```python
from build123d import *

# Parameters (mm, degrees)
BOSS_EXTRUDE1_DEPTH = 9.525
SKETCH1_3_R         = 3.81
BOSS_EXTRUDE2_DEPTH = 2.54
FILLET1_R           = 2.54
SKETCH2_R           = 2.54
CUT_EXTRUDE1_DEPTH  = 106.176870727
SKETCH7_R           = 6.35
CUT_EXTRUDE2_DEPTH  = 18.415
FILLET2_R           = 2.54
FILLET3_R           = 2.54


with BuildPart() as part:
    # Sketch1 → Boss-Extrude1 (new, symmetric)
    with BuildSketch(Plane.XY):
        with BuildLine():
            ThreePointArc((61.722, 65.850540956), (66.416458594, 34.38975697), (39.6875, 17.145))
            Line((39.6875, 17.145), (39.6875, 0))
            Line((39.6875, 0), (79.375, 0))
            Line((79.375, 0), (79.375, 5.461))
            Line((79.375, 5.461), (49.2125, 5.461))
            Line((49.2125, 5.461), (49.2125, 13.012981804))
            ThreePointArc((49.2125, 13.012981804), (67.609880758, 25.71564604), (74.481791773, 46.99))
            ThreePointArc((74.481791773, 46.99), (72.157634164, 58.995640214), (65.823660173, 69.455940354))
            Line((65.823660173, 69.455940354), (61.722, 65.850540956))
        make_face()
        with BuildLine():
            Line((39.6875, 0), (39.6875, 17.145))
            ThreePointArc((39.6875, 17.145), (12.958541406, 34.38975697), (17.653, 65.850540956))
            Line((17.653, 65.850540956), (13.551339827, 69.455940354))
            ThreePointArc((13.551339827, 69.455940354), (7.217365836, 58.995640214), (4.893208227, 46.99))
            ThreePointArc((4.893208227, 46.99), (11.765119242, 25.71564604), (30.1625, 13.012981804))
            Line((30.1625, 13.012981804), (30.1625, 5.461))
            Line((30.1625, 5.461), (0, 5.461))
            Line((0, 5.461), (0, 0))
            Line((0, 0), (39.6875, 0))
        make_face()
    extrude(amount=BOSS_EXTRUDE1_DEPTH, both=True)

    # Sketch1<3> → Boss-Extrude2 (add, symmetric)
    # profile 1 of 2: a face of its own
    with BuildSketch(Plane.XY):
        with BuildLine():
            Line((0, 46.99), (0, 5.461))
            Line((0, 5.461), (30.1625, 5.461))
            Line((30.1625, 5.461), (30.1625, 13.012981804))
            ThreePointArc((30.1625, 13.012981804), (11.765119242, 25.71564604), (4.893208227, 46.99))
            Line((4.893208227, 46.99), (0, 46.99))
        make_face()
        with Locations((8.9535, 17.526)):
            Circle(SKETCH1_3_R, mode=Mode.SUBTRACT)
    # profile 2 of 2: a face of its own
    with BuildSketch(Plane.XY):
        with BuildLine():
            Line((49.2125, 5.461), (79.375, 5.461))
            Line((79.375, 5.461), (79.375, 46.99))
            Line((79.375, 46.99), (74.481791773, 46.99))
            ThreePointArc((74.481791773, 46.99), (67.609880758, 25.71564604), (49.2125, 13.012981804))
            Line((49.2125, 13.012981804), (49.2125, 5.461))
        make_face()
        with Locations((70.4215, 17.526)):
            Circle(SKETCH1_3_R, mode=Mode.SUBTRACT)
    extrude(amount=BOSS_EXTRUDE2_DEPTH, both=True)

    # Fillet1
    fillet1_edges = [part.edges().sort_by_distance(p)[0] for p in [
        (17.653, 65.850540956, 0),
    ]]
    fillet(fillet1_edges, radius=FILLET1_R)
    fillet1_2_edges = [part.edges().sort_by_distance(p)[0] for p in [
        (61.722, 65.850540956, 0),
    ]]
    fillet(fillet1_2_edges, radius=FILLET1_R)
    fillet1_3_edges = [part.edges().sort_by_distance(p)[0] for p in [
        (0, 2.7305, -9.525),
    ]]
    fillet(fillet1_3_edges, radius=FILLET1_R)
    fillet1_4_edges = [part.edges().sort_by_distance(p)[0] for p in [
        (79.375, 2.7305, -9.525),
    ]]
    fillet(fillet1_4_edges, radius=FILLET1_R)
    fillet1_5_edges = [part.edges().sort_by_distance(p)[0] for p in [
        (13.551339827, 69.455940354, 0),
    ]]
    fillet(fillet1_5_edges, radius=FILLET1_R)
    fillet1_6_edges = [part.edges().sort_by_distance(p)[0] for p in [
        (0, 2.7305, 9.525),
    ]]
    fillet(fillet1_6_edges, radius=FILLET1_R)
    fillet1_7_edges = [part.edges().sort_by_distance(p)[0] for p in [
        (79.375, 2.7305, 9.525),
    ]]
    fillet(fillet1_7_edges, radius=FILLET1_R)
    fillet1_8_edges = [part.edges().sort_by_distance(p)[0] for p in [
        (65.823660173, 69.455940354, 0),
    ]]
    fillet(fillet1_8_edges, radius=FILLET1_R)
    fillet1_9_edges = [part.edges().sort_by_distance(p)[0] for p in [
        (79.375, 26.2255, -2.54),
    ]]
    fillet(fillet1_9_edges, radius=FILLET1_R)
    fillet1_10_edges = [part.edges().sort_by_distance(p)[0] for p in [
        (79.375, 26.2255, 2.54),
    ]]
    fillet(fillet1_10_edges, radius=FILLET1_R - 0.0001)  # a hair under: the kernel refuses the full size
    fillet1_11_edges = [part.edges().sort_by_distance(p)[0] for p in [
        (49.2125, 13.012981804, 6.0325),
    ]]
    fillet(fillet1_11_edges, radius=FILLET1_R)
    fillet1_12_edges = [part.edges().sort_by_distance(p)[0] for p in [
        (49.2125, 5.461, 6.0325),
    ]]
    fillet(fillet1_12_edges, radius=FILLET1_R)
    fillet1_13_edges = [part.edges().sort_by_distance(p)[0] for p in [
        (75.658395887, 46.99, -2.54),
    ]]
    fillet(fillet1_13_edges, radius=FILLET1_R - 0.0001)  # a hair under: the kernel refuses the full size

    # Sketch2 → Cut-Extrude1 (cut, through all)
    with BuildSketch(Plane.XZ):
        with Locations(Location((39.6875, 0, 0), (0, 0, 270))):
            Circle(SKETCH2_R)
    extrude(amount=-CUT_EXTRUDE1_DEPTH, mode=Mode.SUBTRACT)

    # Sketch7 → Cut-Extrude2 (cut)
    with BuildSketch(Plane(origin=(0, 19.05, 0), x_dir=(-1, 0, 0), z_dir=(0, -1, 0))):
        with Locations(Location((-39.6875, 0, 0), (0, 0, 270))):
            Circle(SKETCH7_R)
    extrude(amount=CUT_EXTRUDE2_DEPTH, mode=Mode.SUBTRACT)

    # Fillet2
    fillet2_edges = [part.edges().sort_by_distance(p)[0] for p in [
        (30.1625, 5.461, 6.0325),
    ]]
    fillet(fillet2_edges, radius=FILLET2_R)
    fillet2_2_edges = [part.edges().sort_by_distance(p)[0] for p in [
        (30.1625, 13.012981804, 6.0325),
    ]]
    fillet(fillet2_2_edges, radius=FILLET2_R)
    fillet2_3_edges = [part.edges().sort_by_distance(p)[0] for p in [
        (0, 26.2255, 2.54),
    ]]
    fillet(fillet2_3_edges, radius=FILLET2_R)
    fillet2_4_edges = [part.edges().sort_by_distance(p)[0] for p in [
        (0, 26.2255, -2.54),
    ]]
    fillet(fillet2_4_edges, radius=FILLET2_R - 0.0001)  # a hair under: the kernel refuses the full size
    fillet2_5_edges = [part.edges().sort_by_distance(p)[0] for p in [
        (3.716604113, 46.99, 2.54),
    ]]
    fillet(fillet2_5_edges, radius=FILLET2_R - 0.0001)  # a hair under: the kernel refuses the full size

    # Fillet3
    fillet3_edges = [part.edges().sort_by_distance(p)[0] for p in [
        (30.1625, 5.461, -6.0325),
        (30.1625, 13.012981804, -6.0325),
        (49.2125, 13.012981804, -6.0325),
        (49.2125, 5.461, -6.0325),
    ]]
    fillet(fillet3_edges, radius=FILLET3_R)


solid = part.part
```
Read the model definition and answer for the solid it produces. Units are mm, in the model's axes. A direction names the side the tool comes from. Coordinates: 2 decimals unless noted, no trailing zeros. Loops run counter-clockwise (first coordinate to the right, second up) from the corner with the lowest first, then second, coordinate; pieces in that order, holes last. Notation, with made-up numbers: (53, 48.25) -> (86, 48.25) arc R7 cw to (86, 61.25) -> close; hole circle Ø7 at (48.5, -27). An arc over 180 degrees is marked (long way). Return JSON: item names as keys, results as strings.
Item 1: Flat-ended cylindrical pins translate along their axes: P1, Ø3.5, axis at y = 9.5, z = -5.5, coming from the +X side; P2, Ø8, axis at y = 29.5, z = 4, coming from the -X side; P3, Ø3.5, axis at y = 9, z = -5.5, coming from the -X side; P4, Ø10, axis at x = 38, z = -2, coming from the +Y side. Find the tip coordinate at first contact, or state that the pin passes through.
Answers:
{"P1": "stops at x = 49.22", "P2": "stops at x = 0", "P3": "stops at x = 30.05", "P4": "stops at y = 17.92"}
Item 2: For faces 1 (the flat face through (40, 0.635, 3)), 2 (the flat face through (66, 5.461, -6)), 3 (the cylindrical face through (62.7, 65.79, -0.13)), 4 (the cylindrical face through (29.7, 12.61, 6.08)), 5 (the flat face through (66, 17, 2.54)), determine the directions among +Z, -Z, +X, -X, +Y, -Y from which every point of the face is accessible in a straight line to the end or side of a thin tool.
Answers:
{"face 1": "+Y", "face 2": "-Z, +X", "face 3": "+Z, -Z", "face 4": "+Z, -X", "face 5": "+Z, +X"}
Item 3: Find section B-B (x = 36). Determine the outline of the cut face in (y, z) (3 decimals).
Answers:
{"outline": "(0, -9.525) -> (17.378, -9.525) -> (17.378, -5.17) -> (0.635, -5.17) -> (0.635, 5.17) -> (17.378, 5.17) -> (17.378, 9.525) -> (0, 9.525) -> close"}
Item 4: For a pull along Y with two mould halves and no side action, classify faces 6 (the cylindrical face through (33.39, 9.36, -0.83)), 7 (the cylindrical face through (12.588, 18.67, -0.036)), 8 (the cylindrical face through (13.57, 68.33, -0.13)) as +Y half, -Y half, draft (parallel to the pull), parting line (faces both ways), or undercut.
Answers:
{"face 6": "draft", "face 7": "undercut", "face 8": "+Y half"}
Item 5: Find the intervals of material crossed by probe 1 along Y at (x, z) = (63, -7.5); probe 2 along Y at (x, z) = (14, -8); probe 3 along X at (y, z) = (4.75, 0) (1 decimal), in increasing order.
Answers:
{"probe 1": "y = 0 to 5.46, 20.65 to 28.67, 64.34 to 66.77", "probe 2": "y = 0 to 5.46, 23.01 to 32.31, 60.65 to 68.34", "probe 3": "x = 0 to 33.3, 46 to 79.4"}
